Check sheet for the modelled part. Datum: model origin and axes. Units: mm. A direction names the side the tool comes from. Coordinates: 2 decimals unless noted, no trailing zeros. Loops run counter-clockwise (first coordinate to the right, second up) from the corner with the lowest first, then second, coordinate; pieces in that order, holes last. Notation, with made-up numbers: (11.25, 62) - (49.25, 62) arc R14 ccw to (49.25, 73) - close; hole circle Ø9 at (51, 68.5). An arc over 180 degrees is marked (long way). Use a Markdown table: item, result. Add a question column.
1) Sectioned sample at D-D, the plane z = 11. Enter the section's corners in (x, y).
2) Draft check along Y on faces 1 (the flat face through (48, 12, 20)), 2 (the flat face through (-25, 2.5, -12)), 3 (the flat face through (50, 0, 0)). Enter one of: pulls with the +Y half, pulls with the -Y half, needs draft (parallel to the pull), parting line crosses it, or undercut.
3) Tool access check on faces 4 (the flat face through (-48, 12, 5)), 5 (the flat face through (-30, 5.5, -6)), 6 (the cylindrical face through (-49, -2.5, 13.9)), 7 (the flat face through (30, -4, -3.5)), 8 (the flat face through (-25, 5.5, -13)). Record the directions out of +Z, -Z, +X, -X, +Y, -Y that give a thin tool (end or side, any length) a straight path to the whole face; none if there is none.
4) Sectioned sample at B-B, the plane x = -23. Enter the section's corners in (y, z), then the cut area to 3 significant figures.
5) Sectioned sample at A-A, the plane z = 1. Enter the section's corners in (x, y), then the cut area to 4 significant figures.
6) Go/stop test with flat-tipped pins: P1, Ø10, axis at x = -33.5, z = -5.5, coming from the +Y side; P2, Ø3.5, axis at y = 11, z = 4, coming from the +X side; P3, Ø4, axis at x = -34, y = -5, coming from the +Z side; P4, Ø1, axis at x = 34, y = 7.5, coming from the +Z side. Record where each tip stops, or that it passes through.
7) Thickness scan on line 1 (X direction, y = -2, z = -16); line 2 (X direction, y = 0.75, z = -10); line 3 (Z direction, x = -9, y = 6.25). Record the ranges inside material, lowest first.
8) Sectioned sample at C-C, the plane z = -13.5. State how many separate pieces and enclosed holes the cut face has, then the cut area to 3 significant figures.
from build123d import *

# Parameters (mm, degrees)
SKETCH1_W                  = 45
SKETCH1_H                  = 15
BOSS_EXTRUDE1_DEPTH        = 50
SKETCH2_W                  = 96
SKETCH2_H                  = 26
CUT_EXTRUDE1_DEPTH         = 13
SHELL1_START               = -48
SHELL1_OUTLINE_W           = 11
SHELL1_OUTLINE_H           = 17
SHELL1_DEPTH               = 96
SKETCH3_W                  = 20
SKETCH3_H                  = 10
CUT_EXTRUDE2_DEPTH         = 2
LPATTERN1_COUNT            = 2
LPATTERN1_PITCH            = 30
LPATTERN1_COL_COUNT        = 2
LPATTERN1_COL_PITCH        = 30
BOSS_EXTRUDE2_REACH        = 68.372
SKETCH4_W                  = 12
SKETCH4_H                  = 4
SKETCH4_W_2                = 2
SKETCH4_H_2                = 3
SKETCH5_W                  = 12
SKETCH5_H                  = 1.5
BOSS_EXTRUDE3_DEPTH        = 7
CHAMFER1_SIZE              = 0.5
FILLET1_R                  = 2
LPATTERN2_COUNT            = 3
LPATTERN2_PITCH            = 30
CHAMFER1_OF_LPATTERN2_SIZE = 0.5
FILLET1_OF_LPATTERN2_R     = 2
SKETCH6_W                  = 3
SKETCH6_H                  = 3
BOSS_EXTRUDE4_DEPTH        = 1.25
BOSS_EXTRUDE4_2_DEPTH      = 1.25
BOSS_EXTRUDE5_DEPTH        = 0.5
SKETCH8_W                  = 7.5
SKETCH8_H                  = 5
BOSS_EXTRUDE6_DEPTH        = 0.5
CHAMFER2_SIZE              = 0.5
CHAMFER4_SIZE              = 1.25
CHAMFER2_OF_MIRROR7_SIZE   = 0.5
CHAMFER4_OF_MIRROR7_SIZE   = 1.25
CUT_EXTRUDE3_DEPTH         = 2


# Read off the part's stored shape, not the designer's step: Shell1
with BuildPart() as part:
    # Sketch1 → Boss-Extrude1 (new, symmetric)
    with BuildSketch(Plane(origin=(0, 0, 0), x_dir=(0, 0, -1), z_dir=(1, 0, 0))):
        Rectangle(SKETCH1_W, SKETCH1_H)
    extrude(amount=BOSS_EXTRUDE1_DEPTH, both=True)

    # Sketch2 → Cut-Extrude1 (cut)
    with BuildSketch(Plane(origin=(0, 7.5, 0), x_dir=(1, 0, 0), z_dir=(0, 1, 0))):
        with Locations((0, -9.5)):
            Rectangle(SKETCH2_W, SKETCH2_H)
    extrude(amount=-CUT_EXTRUDE1_DEPTH, mode=Mode.SUBTRACT)

    # Shell1 outline → Shell1 (cut)
    with BuildSketch(Plane.YZ.offset(SHELL1_START)):
        with Locations((0, -12)):
            Rectangle(SHELL1_OUTLINE_W, SHELL1_OUTLINE_H)
    extrude(amount=SHELL1_DEPTH, mode=Mode.SUBTRACT)

    # Sketch3 → Cut-Extrude2 (cut)
    with BuildSketch(Plane(origin=(0, 7.5, 0), x_dir=(1, 0, 0), z_dir=(0, 1, 0))):
        with Locations((0, 13)):
            Rectangle(SKETCH3_W, SKETCH3_H)
    cut_extrude2 = extrude(amount=-CUT_EXTRUDE2_DEPTH, mode=Mode.SUBTRACT)

    # LPattern1: Cut-Extrude2 ×2
    with Locations(*[(-i * LPATTERN1_PITCH, 0, 0) for i in range(1, LPATTERN1_COUNT)]):
        add(cut_extrude2, mode=Mode.SUBTRACT)

    # LPattern1 col: Cut-Extrude2 ×2
    with Locations(*[(i * LPATTERN1_COL_PITCH, 0, 0) for i in range(1, LPATTERN1_COL_COUNT)]):
        add(cut_extrude2, mode=Mode.SUBTRACT)

    # Boss-Extrude2: up to this face of the body (flat: up to its plane)
    boss_extrude2_end = Plane(part.part.faces().sort_by_distance((0, 6.5, -3.5))[0])
    # Sketch4 → Boss-Extrude2 (add, up to the picked face)
    with BuildSketch(Plane.XY.offset(-20.5), mode=Mode.PRIVATE) as boss_extrude2_sk1:
        with Locations((-30, -3.5)):
            Rectangle(SKETCH4_W, SKETCH4_H)
    boss_extrude2_tool1 = split(extrude(boss_extrude2_sk1.sketch, amount=BOSS_EXTRUDE2_REACH, mode=Mode.PRIVATE), bisect_by=boss_extrude2_end, keep=Keep.BOTH, mode=Mode.PRIVATE)
    # Sketch4 → Boss-Extrude2 (add, up to the picked face)
    with BuildSketch(Plane.XY.offset(-20.5), mode=Mode.PRIVATE) as boss_extrude2_sk2:
        with Locations((-35, 4)):
            Rectangle(SKETCH4_W_2, SKETCH4_H_2)
    boss_extrude2_tool2 = split(extrude(boss_extrude2_sk2.sketch, amount=BOSS_EXTRUDE2_REACH, mode=Mode.PRIVATE), bisect_by=boss_extrude2_end, keep=Keep.BOTH, mode=Mode.PRIVATE)
    # Sketch4 → Boss-Extrude2 (add, up to the picked face)
    with BuildSketch(Plane.XY.offset(-20.5), mode=Mode.PRIVATE) as boss_extrude2_sk3:
        with Locations((-25, 4)):
            Rectangle(SKETCH4_W_2, SKETCH4_H_2)
    boss_extrude2_tool3 = split(extrude(boss_extrude2_sk3.sketch, amount=BOSS_EXTRUDE2_REACH, mode=Mode.PRIVATE), bisect_by=boss_extrude2_end, keep=Keep.BOTH, mode=Mode.PRIVATE)
    boss_extrude2_1 = boss_extrude2_tool1.solids().sort_by(Axis((-30, -3.5, -20.5), (0, 0, 1)))[0]
    add(boss_extrude2_1)
    boss_extrude2_2 = boss_extrude2_tool2.solids().sort_by(Axis((-35, 4, -20.5), (0, 0, 1)))[0]
    add(boss_extrude2_2)
    boss_extrude2_3 = boss_extrude2_tool3.solids().sort_by(Axis((-25, 4, -20.5), (0, 0, 1)))[0]
    add(boss_extrude2_3)
    boss_extrude2 = boss_extrude2_1 + boss_extrude2_2 + boss_extrude2_3  # Boss-Extrude2 as one shape, for the pattern or mirror that repeats it

    # Sketch5 → Boss-Extrude3 (add)
    with BuildSketch(Plane(origin=(0, -1.5, 0), x_dir=(1, 0, 0), z_dir=(0, 1, 0))):
        with Locations((-30, 19.75)):
            Rectangle(SKETCH5_W, SKETCH5_H)
    boss_extrude3 = extrude(amount=BOSS_EXTRUDE3_DEPTH)

    # Chamfer1
    chamfer1_edges = [part.edges().sort_by_distance(p)[0] for p in [
        (-35, 2.5, -3.5),
        (-25, 2.5, -3.5),
        (-30, -1.5, -3.5),
    ]]
    chamfer(chamfer1_edges, length=CHAMFER1_SIZE)

    # Fillet1
    fillet1_edges = [part.edges().sort_by_distance(p)[0] for p in [
        (-24, -5.5, -12),
        (-36, -5.5, -12),
    ]]
    fillet(fillet1_edges, radius=FILLET1_R)

    # LPattern2: Boss-Extrude2, Boss-Extrude3 ×3
    with Locations(*[(i * LPATTERN2_PITCH, 0, 0) for i in range(1, LPATTERN2_COUNT)]):
        add(boss_extrude2)
        add(boss_extrude3)

    # Chamfer1 of LPattern2
    chamfer1_of_lpattern2_edges = [part.edges().sort_by_distance(p)[0] for p in [
        (-5, 2.5, -3.5),
        (5, 2.5, -3.5),
        (0, -1.5, -3.5),
        (25, 2.5, -3.5),
        (35, 2.5, -3.5),
        (30, -1.5, -3.5),
    ]]
    chamfer(chamfer1_of_lpattern2_edges, length=CHAMFER1_OF_LPATTERN2_SIZE)

    # Fillet1 of LPattern2
    fillet1_of_lpattern2_edges = [part.edges().sort_by_distance(p)[0] for p in [
        (6, -5.5, -12),
        (-6, -5.5, -12),
        (36, -5.5, -12),
        (24, -5.5, -12),
    ]]
    fillet(fillet1_of_lpattern2_edges, radius=FILLET1_OF_LPATTERN2_R)



with BuildPart() as body_2:
    # Sketch6 → Boss-Extrude4 (new body)
    with BuildSketch(Plane.ZY.offset(-48)):
        with Locations((19.5, 10.5)):
            Rectangle(SKETCH6_W, SKETCH6_H)
    boss_extrude4 = extrude(amount=-BOSS_EXTRUDE4_DEPTH)



with BuildPart() as body_3:
    # Sketch6 → Boss-Extrude4 2 (new body)
    with BuildSketch(Plane.ZY.offset(-48)):
        with Locations((4.5, 10.5)):
            Rectangle(SKETCH6_W, SKETCH6_H)
    boss_extrude4_2 = extrude(amount=-BOSS_EXTRUDE4_2_DEPTH)


with BuildPart() as body_2_1:
    add(body_2.part)

    add(body_3.part)  # Boss-Extrude5 merges body 3
    # Sketch7 → Boss-Extrude5 (add)
    with BuildSketch(Plane.ZY.offset(-48)):
        Polygon((18, 12), (13.5, 7.5), (21, 7.5), (21, 12), align=None)
        Polygon((3, 12), (-1.5, 7.5), (6, 7.5), (6, 12), align=None)
    boss_extrude5 = extrude(amount=BOSS_EXTRUDE5_DEPTH)


with BuildPart() as part_1:
    add(part.part)

    add(body_2_1.part)  # Boss-Extrude6 merges body 2
    # Sketch8 → Boss-Extrude6 (add)
    with BuildSketch(Plane.ZY.offset(-47.5)):
        with Locations((2.25, 5)):
            Rectangle(SKETCH8_W, SKETCH8_H)
        with Locations((17.25, 5)):
            Rectangle(SKETCH8_W, SKETCH8_H)
    boss_extrude6 = extrude(amount=-BOSS_EXTRUDE6_DEPTH)

    # Chamfer2
    chamfer2_edges = [part_1.edges().sort_by_distance(p)[0] for p in [
        (47.5, 5, -1.5),
        (47.5, 5, 13.5),
    ]]
    chamfer(chamfer2_edges, length=CHAMFER2_SIZE - 0.0001)  # a hair under: the kernel refuses the full size

    # Chamfer4
    chamfer4_edges = [part_1.edges().sort_by_distance(p)[0] for p in [
        (49.25, 10.5, 3),
        (49.25, 10.5, 18),
    ]]
    chamfer(chamfer4_edges, length=CHAMFER4_SIZE - 0.0001)  # a hair under: the kernel refuses the full size

    # Mirror7: Boss-Extrude4, Boss-Extrude4 2, Boss-Extrude5, Boss-Extrude6 across plane
    add(boss_extrude4.mirror(Plane(origin=(0, 0, 0), x_dir=(0, 0, 1), z_dir=(1, 0, 0))))
    add(boss_extrude4_2.mirror(Plane(origin=(0, 0, 0), x_dir=(0, 0, 1), z_dir=(1, 0, 0))))
    add(boss_extrude5.mirror(Plane(origin=(0, 0, 0), x_dir=(0, 0, 1), z_dir=(1, 0, 0))))
    add(boss_extrude6.mirror(Plane(origin=(0, 0, 0), x_dir=(0, 0, 1), z_dir=(1, 0, 0))))

    # Chamfer2 of Mirror7
    chamfer2_of_mirror7_edges = [part_1.edges().sort_by_distance(p)[0] for p in [
        (-47.5, 5, -1.5),
        (-47.5, 5, 13.5),
    ]]
    chamfer(chamfer2_of_mirror7_edges, length=CHAMFER2_OF_MIRROR7_SIZE - 0.0001)  # a hair under: the kernel refuses the full size

    # Chamfer4 of Mirror7
    chamfer4_of_mirror7_edges = [part_1.edges().sort_by_distance(p)[0] for p in [
        (-49.25, 10.5, 3),
        (-49.25, 10.5, 18),
    ]]
    chamfer(chamfer4_of_mirror7_edges, length=CHAMFER4_OF_MIRROR7_SIZE - 0.0001)  # a hair under: the kernel refuses the full size

    # Sketch10 → Cut-Extrude3 (cut)
    with BuildSketch(Plane.ZY.offset(50)):
        with BuildLine():
            Line((19, -4.6), (16, -4.6))
            ThreePointArc((16, -4.6), (13.9, -2.5), (16, -0.4))
            Line((16, -0.4), (19, -0.4))
            ThreePointArc((19, -0.4), (21.1, -2.5), (19, -4.6))
        make_face()
    extrude(amount=-CUT_EXTRUDE3_DEPTH, mode=Mode.SUBTRACT)


solid = part_1.part
Solved:
| question | item | result |
|---|---|---|
| 1 | outline | (-50, -7.5) - (50, -7.5) - (50, 7.5) - (48, 7.5) - (48, -5.5) - (-48, -5.5) - (-48, 7.5) - (-50, 7.5) - close |
| 2 | face 1 | pulls with the +Y half |
| 2 | face 2 | undercut |
| 2 | face 3 | needs draft |
| 3 | face 4 | +Z, -Z, +X, -X, +Y |
| 3 | face 5 | +Z |
| 3 | face 6 | -X |
| 3 | face 7 | +Z, +Y |
| 3 | face 8 | +Y |
| 4 | outline | (-7.5, -22.5) - (7.5, -22.5) - (7.5, -18) - (5.5, -18) - (5.5, -20.5) - (-5.23, -20.5) - (-5.23, -3.5) - (-5.5, -3.5) - (-5.5, 22.5) - (-7.5, 22.5) - close; (5.5, -8) - (7.5, -8) - (7.5, -3.5) - (5.5, -3.5) - close |
| 4 | area | 135 mm2 |
| 5 | outline | (-50, -7.5) - (50, -7.5) - (50, 7.5) - (48, 7.5) - (48, 10) - (47.5, 10) - (47.5, 2.5) - (48, 2.5) - (48, -5.5) - (-48, -5.5) - (-48, 2.5) - (-47.5, 2.5) - (-47.5, 10) - (-48, 10) - (-48, 7.5) - (-50, 7.5) - close |
| 5 | area | 259.5 mm2 |
| 6 | P1 | stops at y = 7.5 |
| 6 | P2 | stops at x = 49.25 |
| 6 | P3 | stops at z = 22.5 |
| 6 | P4 | stops at z = -3.5 |
| 7 | line 1 | x = -50 to -48, -36 to -24, -6 to 6, 24 to 36, 48 to 50 |
| 7 | line 2 | x = -50 to -48, 48 to 50 |
| 7 | line 3 | z = -22.5 to -18, -8 to -3.5 |
| 8 | separate pieces | 9 |
| 8 | enclosed holes | 0 |
| 8 | area | 509 mm2 |
